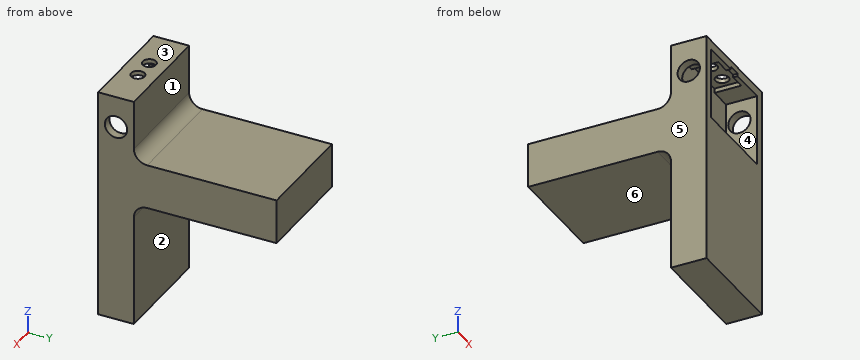
```python
from build123d import *

# Parameters (mm, degrees)
ESQUISSE1_W                  = 120
ESQUISSE1_H                  = 200
BOSS_EXTRU_2_DEPTH           = 25
ESQUISSE3_W                  = 120
ESQUISSE3_H                  = 40
BOSS_EXTRU_3_DEPTH           = 70
CONG_1_R                     = 15
ESQUISSE4_W                  = 120
ESQUISSE4_H                  = 40
BOSS_EXTRU_4_DEPTH           = 140
CONG_2_R                     = 15
ESQUISSE5_W                  = 50
ESQUISSE5_H                  = 30
BOSS_EXTRU_9_DEPTH           = 7.5
ESQUISSE7_W                  = 100
ESQUISSE7_H                  = 80
ENL_V_MAT_EXTRU_1_DEPTH      = 35
ENL_V_MAT_EXTRU_7_REACH      = 351.285
ESQUISSE8_R                  = 7.5
ESQUISSE12_W                 = 50
ESQUISSE12_H                 = 30
ENL_V_MAT_EXTRU_8_DEPTH      = 5
ENL_V_MAT_EXTRU_9_DEPTH      = 286.700892543
ENL_V_MAT_EXTRU_9_DEPTH_BACK = 286.700892543
ESQUISSE13_R                 = 12.5
ESQUISSE14_W                 = 15
ESQUISSE14_H                 = 5
ENL_V_MAT_EXTRU_10_DEPTH     = 3


with BuildPart() as part:
    # Esquisse1 → Boss.-Extru.2 (new, symmetric)
    with BuildSketch(Plane.XY):
        with Locations((60, 100)):
            Rectangle(ESQUISSE1_W, ESQUISSE1_H)
    extrude(amount=BOSS_EXTRU_2_DEPTH, both=True)

    # Esquisse3 → Boss.-Extru.3 (add)
    with BuildSketch(Plane.XY.offset(25)):
        with Locations((60, 20)):
            Rectangle(ESQUISSE3_W, ESQUISSE3_H)
    extrude(amount=BOSS_EXTRU_3_DEPTH)

    # Congé1
    cong_1_edges = [part.edges().sort_by_distance(p)[0] for p in [
        (60, 40, 25),
    ]]
    fillet(cong_1_edges, radius=CONG_1_R)

    # Esquisse4 → Boss.-Extru.4 (add)
    with BuildSketch(Plane(origin=(0, 0, -25), x_dir=(-1, 0, 0), z_dir=(0, 0, -1))):
        with Locations((-60, 20)):
            Rectangle(ESQUISSE4_W, ESQUISSE4_H)
    extrude(amount=BOSS_EXTRU_4_DEPTH)

    # Congé2
    cong_2_edges = [part.edges().sort_by_distance(p)[0] for p in [
        (60, 40, -25),
    ]]
    fillet(cong_2_edges, radius=CONG_2_R)

    # Esquisse5 → Boss.-Extru.9 (add)
    with BuildSketch(Plane.XY.offset(95)):
        with Locations((60, 20)):
            Rectangle(ESQUISSE5_W, ESQUISSE5_H)
    extrude(amount=-BOSS_EXTRU_9_DEPTH)

    # Esquisse7 → Enlèv. mat.-Extru.1 (cut)
    with BuildSketch(Plane.XZ):
        with Locations((60, 45)):
            Rectangle(ESQUISSE7_W, ESQUISSE7_H)
    extrude(amount=-ENL_V_MAT_EXTRU_1_DEPTH, mode=Mode.SUBTRACT)

    # Esquisse8 → Enlèv. mat.-Extru.7 (cut, up to next)
    with BuildSketch(Plane.XY.offset(95), mode=Mode.PRIVATE) as enl_v_mat_extru_7_sk1:
        with Locations((47.5, 20)):
            Circle(ESQUISSE8_R)
    enl_v_mat_extru_7_tool1 = extrude(enl_v_mat_extru_7_sk1.sketch, amount=-ENL_V_MAT_EXTRU_7_REACH, mode=Mode.PRIVATE) & part.part
    # Esquisse8 → Enlèv. mat.-Extru.7 (cut, up to next)
    with BuildSketch(Plane.XY.offset(95), mode=Mode.PRIVATE) as enl_v_mat_extru_7_sk2:
        with Locations((72.5, 20)):
            Circle(ESQUISSE8_R)
    enl_v_mat_extru_7_tool2 = extrude(enl_v_mat_extru_7_sk2.sketch, amount=-ENL_V_MAT_EXTRU_7_REACH, mode=Mode.PRIVATE) & part.part
    add(enl_v_mat_extru_7_tool1.solids().sort_by_distance((47.5, 20, 95))[0], mode=Mode.SUBTRACT)
    add(enl_v_mat_extru_7_tool2.solids().sort_by_distance((72.5, 20, 95))[0], mode=Mode.SUBTRACT)

    # Esquisse12 → Enlèv. mat.-Extru.8 (cut)
    with BuildSketch(Plane(origin=(0, 0, 85), x_dir=(-1, 0, 0), z_dir=(0, 0, -1))):
        with Locations((-60, 20)):
            Rectangle(ESQUISSE12_W, ESQUISSE12_H)
    extrude(amount=-ENL_V_MAT_EXTRU_8_DEPTH, mode=Mode.SUBTRACT)

    # Esquisse13 → Enlèv. mat.-Extru.9 (cut, two sides: drawn at the far end of the back side and taken through both)
    with BuildSketch(Plane(origin=(120, 0, 0), x_dir=(0, 0, -1), z_dir=(1, 0, 0)).offset(-ENL_V_MAT_EXTRU_9_DEPTH_BACK)):
        with Locations((-60, 20)):
            Circle(ESQUISSE13_R)
    extrude(amount=ENL_V_MAT_EXTRU_9_DEPTH + ENL_V_MAT_EXTRU_9_DEPTH_BACK, mode=Mode.SUBTRACT)

    # Esquisse14 → Enlèv. mat.-Extru.10 (cut)
    with BuildSketch(Plane(origin=(0, 0, 85), x_dir=(-1, 0, 0), z_dir=(0, 0, -1))):
        with Locations((-60, 2.5)):
            Rectangle(ESQUISSE14_W, ESQUISSE14_H)
    extrude(amount=-ENL_V_MAT_EXTRU_10_DEPTH, mode=Mode.SUBTRACT)


solid = part.part
```
CAD build for the part. Positions are in the model's coordinates, mm. Face numbers are marked on the shaded views. A direction names the side the tool comes from. Coordinates: 2 decimals unless noted, no trailing zeros. Write each loop counter-clockwise with the first axis right and the second up, starting at its lowest first coordinate (ties: lowest second). Pieces come first, ordered by that corner, then holes. Notation, with made-up numbers: (-32.5, 28.5) -> (13.5, 28.5) arc R14 ccw to (13.5, 36.5) -> close; hole circle Ø11 at (12.5, 1.25). An arc over 180 degrees is marked (long way). Return JSON: item names as keys, results as strings. Group by question number.
Q1. Pull direction X, two halves, no side cores. Call the marked faces 4, 5 and 6: released by +X, released by -X, zero draft, split by the parting line, or undercut.
Q2. Cut at B-B, the plane z = 60. Give the cut face in (x, y).
Q3. Which spindle directions (+Z, -Z, +X, -X, +Y, -Y) get a long thin tool onto all of the face, cutting with end or side? Do the marked faces 1, 2 and 3. Say none if no direction does.
Q4. Cut at A-A, the plane y = 20. Give the cut face in (x, z).
Q5. Cut at C-C, the plane x = 72.5. Give the cut face in (y, z).
Q6. Drill centre lines: line 1 (Z direction, x = 5, y = 20); line 2 (Y direction, x = 5, z = 60); line 3 (Y direction, x = 72.5, z = 91.85). Where is each one in solid material? Low to high.
Q7. Flat gauge pins, fed straight in: pin 1 (1.5 mm diameter, centred on y = 18, z = 87, fed in from -X); pin 2 (6 mm diameter, centred on x = 90.5, z = 50, fed in from -Y); pin 3 (8 mm diameter, centred on x = 60, y = 92, fed in from +Z); pin 4 (5.5 mm diameter, centred on x = 53.5, z = 87.5, fed in from +Y). Where does each tip first touch, or does it go through?
Q8. Cut at D-D, the plane z = 13. Give the cut face in (x, y).
Returned:
{
 "1": {"face 4": "undercut", "face 5": "released by -X", "face 6": "zero draft"},
 "2": {"outline": "(0, 0) -> (10, 0) -> (10, 7.5) -> (0, 7.5) -> close; (0, 32.5) -> (10, 32.5) -> (10, 35) -> (110, 35) -> (110, 32.5) -> (120, 32.5) -> (120, 40) -> (0, 40) -> close; (110, 0) -> (120, 0) -> (120, 7.5) -> (110, 7.5) -> close"},
 "3": {"face 1": "+Z, +X, -X, +Y", "face 2": "-Z, +X, -X, +Y", "face 3": "+Z, +X, -X, +Y, -Y"},
 "4": {"outline": "(0, -165) -> (120, -165) -> (120, 47.5) -> (110, 47.5) -> (110, 5) -> (10, 5) -> (10, 47.5) -> (0, 47.5) -> close; (0, 72.5) -> (10, 72.5) -> (10, 85) -> (35, 85) -> (35, 90) -> (40, 90) -> (40, 95) -> (0, 95) -> close; (55, 90) -> (65, 90) -> (65, 95) -> (55, 95) -> close; (80, 90) -> (85, 90) -> (85, 85) -> (110, 85) -> (110, 72.5) -> (120, 72.5) -> (120, 95) -> (80, 95) -> close"},
 "5": {"outline": "(0, -165) -> (40, -165) -> (40, -40) arc R15 cw to (55, -25) -> (200, -25) -> (200, 25) -> (55, 25) arc R15 cw to (40, 40) -> (40, 95) -> (27.5, 95) -> (27.5, 90) -> (35, 90) -> (35, 5) -> (0, 5) -> close; (0, 85) -> (5, 85) -> (5, 90) -> (12.5, 90) -> (12.5, 95) -> (0, 95) -> close"},
 "6": {"line 1": "z = -165 to 47.5, 72.5 to 95", "line 2": "y = 0 to 7.5, 32.5 to 40", "line 3": "y = 0 to 12.5, 27.5 to 40"},
 "7": {"pin 1": "stops at x = 0", "pin 2": "stops at y = 35", "pin 3": "stops at z = 25", "pin 4": "stops at y = 40"},
 "8": {"outline": "(0, 0) -> (10, 0) -> (10, 35) -> (110, 35) -> (110, 0) -> (120, 0) -> (120, 200) -> (0, 200) -> close"}
}
